Check sheet for the modelled part. Datum: model origin and axes. Units: mm. A direction names the side the tool comes from. Coordinates: 2 decimals unless noted, no trailing zeros. Write each loop counter-clockwise with the first axis right and the second up, starting at its lowest first coordinate (ties: lowest second). Pieces come first, ordered by that corner, then holes. Notation, with made-up numbers: M 5.25,3.25 L 63.25,3.25 A19 cw 63.25,36.25 Z; hole C 39,22 d1. An arc over 180 degrees is marked long. Answer as CSV lines item,"result". Start each with the question number.
1) Section check C-C (z = -18.5). Record the cut outline in (x, y).
2) Draft check along Y on faces 4 (the cylindrical face through (-0.189, -4.296, -27.779)), 5 (the conical face through (5.2, -1.2, -23)), 6 (the conical face through (4.3, -1, -22.8)), 7 (the flat face through (4, -2, -32.696)). Enter one of: +Y half, -Y half, draft (parallel to the pull), parting line (faces both ways), or undercut.
3) Go/stop test with flat-tipped pins: pin 1 Ø1.5 at (x, y) = (3.5, 5.5) entering from -Z; pin 2 Ø4 at (x, y) = (-0.5, 3) entering from -Z; pin 3 Ø1 at (y, z) = (-2, -4.5) entering from -X; pin 4 Ø6 at (y, z) = (1.5, -25) entering from -X. Record where each tip stops, or that it passes through.
4) Access from +Z, -Z, +X, -X, +Y, -Y to the whole of each face (thin tool, end or side, straight path). Record for faces 1 (the cylindrical face through (1.9, 5.9, -9.5)), 2 (the cylindrical face through (6.616, -0.737, -3.23)), 3 (the cylindrical face through (-5.156, -0.677, -27.901)).
5) Material ranges on L1, parallel to X at y = 0.25, z = -16; L2, parallel to X at y = -0.25, z = -28.5, recorded low to high. Write a range as [from, to].
6) Section check A-A (y = 0). Record the cut outline in (x, z).
Autodesk Inventor part; units mm, degrees
ref_plane "XZ Plane" through (0, 0, 0) normal (0, 1, 0) x (-1, 0, 0)
ref_plane "XY Plane" through (0, 0, 0) normal (0, 0, 1) x (1, 0, 0)
sketch "Sketch1" plane through (0, 0, 0) normal (1, 0, 0) x (0, 1, 0)
  line L0 (6.2, 1.0944) -> (6.2, -19.7056)
  line L1 (4.3, -32.6965) -> (4.3, -22.9965)
  line L2 (6.2, -19.7056) -> (4.3, -22.9965)
  line L3 (7.1, -19.9467) -> (7.1, 1.0944)
  line L4 (5.2, -32.6965) -> (5.2, -23.2376)
  line L5 (5.2, -23.2376) -> (7.1, -19.9467)
  line L6 (6.2, 1.0944) -> (7.1, 1.0944)
  line L7 (4.3, -32.6965) -> (5.2, -32.6965)
  line L8 (0, 0) -> (0, -7.1245) construction
  dimension "d5" = 6.2
  dimension "d6" = 4.3
  dimension "d7" = 0.9
  dimension "d8" = 0.9
  dimension "d9" = 0.9
  dimension "d10" = 20.8
  dimension "d11" = 9.7
  dimension "d12" = 150
revolve "Revolution1" add sketch "Sketch1" angle 360 about axis through (0, 0, 0) along (0, 0, -1)
ref_plane "Work Plane1" through (8, 0, 0) normal (1, 0, 0) x (0, 1, 0)
sketch "Sketch2" plane through (8, 0, 0) normal (1, 0, 0) x (0, 1, 0)
  line L0 (0, 1.0944) -> (0, -3.9056) construction
  circle A0 centre (0, -3.9056) radius 1
  point P0 (0, 0)
  dimension "d15" = 5
  dimension "d16" = 2
extrude "Extrusion1" cut sketch "Sketch2" against normal blind 10
pattern_circular "Circular Pattern1" count 4 over 360 about axis through (0, 0, -21.351) along (0, 0, -1) of "Extrusion1"
properties part number "fuel"
Results found:
1,outline,"C 0,0 d14.2; hole C 0,0 d12.4"
2,face 4,"undercut"
2,face 5,"parting line"
2,face 6,"undercut"
2,face 7,"draft"
3,pin 1,"stops at z = -22.25"
3,pin 2,"stops at z = -32.7"
3,pin 3,"stops at x = -6.94"
3,pin 4,"stops at x = -5.81"
4,face 1,"+Z"
4,face 2,"+X, -X"
4,face 3,"-Z"
5,L1,"x = [-7.1, -6.19], [6.19, 7.1]"
5,L2,"x = [-5.19, -4.29], [4.29, 5.19]"
6,outline,"M -7.1,-19.95 L -5.2,-23.24 L -5.2,-32.7 L -4.3,-32.7 L -4.3,-23 L -6.2,-19.71 L -6.2,-4.91 L -7.1,-4.91 Z; M -7.1,-2.91 L -6.2,-2.91 L -6.2,1.09 L -7.1,1.09 Z; M 4.3,-32.7 L 5.2,-32.7 L 5.2,-23.24 L 7.1,-19.95 L 7.1,-4.91 L 6.2,-4.91 L 6.2,-19.71 L 4.3,-23 Z; M 6.2,-2.91 L 7.1,-2.91 L 7.1,1.09 L 6.2,1.09 Z"
